Input: part model. Units: mm. Frame: model coordinates. A direction names the side the tool comes from. Coordinates: 2 decimals unless noted, no trailing zeros. Write each loop counter-clockwise with the first axis right and the second up, starting at its lowest first coordinate (ties: lowest second). Pieces come first, ordered by that corner, then holes. Notation, with made-up numbers: (36, 85.5) - (93, 85.5) arc R33 cw to (93, 121.5) - close; hole circle Ø8 at (60.5, 28.5). An arc over 180 degrees is marked (long way). Use CSV: the item, a comma, the result in double quotes.
```python
from build123d import *

# Parameters (mm, degrees)
SKETCH_2_W          = 85.8
SKETCH_2_H          = 85.8
SKETCH_2_R          = 6
EXTRUDE_1_DEPTH     = 13.5
FILLET_1_R          = 10
SKETCH_3_R          = 10
CUT_EXTRUDE_1_DEPTH = 65.366683929


with BuildPart() as part:
    # 草图1 → 旋转1 (revolve)
    with BuildSketch(Plane.XY, mode=Mode.PRIVATE) as revolve_1_sk:
        Polygon((10, 30), (14.5, 30), (14.5, 20), (23, 20), (23, 21.5), (28, 21.5), (28, 3.5), (14.5, 3.5), (14.5, 0), (10, 0), align=None)
    revolve(revolve_1_sk.sketch.rotate(Axis((0, 50.942477876, 0), (0, -1, 0)), 90), axis=Axis((0, 50.942477876, 0), (0, -1, 0)))

    # 草图2 → 凸台-拉伸1 (add)
    with BuildSketch(Plane(origin=(0, -5, 0), x_dir=(1, 0, 0), z_dir=(0, 1, 0))):
        Rectangle(SKETCH_2_W, SKETCH_2_H)
        with Locations(Location((-31.75, 31.75, 0), (0, 0, 270))):
            Circle(SKETCH_2_R, mode=Mode.SUBTRACT)
        with Locations(Location((31.75, 31.75, 0), (0, 0, 270))):
            Circle(SKETCH_2_R, mode=Mode.SUBTRACT)
        with Locations(Location((31.75, -31.75, 0), (0, 0, 270))):
            Circle(SKETCH_2_R, mode=Mode.SUBTRACT)
        with Locations(Location((-31.75, -31.75, 0), (0, 0, 270))):
            Circle(SKETCH_2_R, mode=Mode.SUBTRACT)
    extrude(amount=EXTRUDE_1_DEPTH)

    # 圆角1
    fillet_1_edges = [part.edges().sort_by_distance(p)[0] for p in [
        (42.9, 1.75, 42.9),
        (42.9, 1.75, -42.9),
        (-42.9, 1.75, -42.9),
        (-42.9, 1.75, 42.9),
    ]]
    fillet(fillet_1_edges, radius=FILLET_1_R)

    # 草图3 → 切除-拉伸1 (cut, through all)
    with BuildSketch(Plane(origin=(0, 8.5, 0), x_dir=(1, 0, 0), z_dir=(0, 1, 0))):
        with Locations(Location((0, 0, 0), (0, 0, 270))):
            Circle(SKETCH_3_R)
    extrude(amount=-CUT_EXTRUDE_1_DEPTH, mode=Mode.SUBTRACT)


solid = part.part
```
(1) Pin query (flat end, axial travel): pin 1 Ø1.5 at (y, z) = (18.5, 12.5) entering from +X; pin 2 Ø3 at (y, z) = (21, -2) entering from -X; pin 3 Ø15.5 at (x, z) = (31.75, 31.75) entering from +Y. Return the tip coordinate at first contact, or that it passes through.
Check values:
pin 1,"x = 25.42"
pin 2,"x = -28"
pin 3,"y = 8.5"
(2) Cut plane C-C on x = -31.75. Return loops of the section in (y, z).
Check values:
outline,"(-5, -42.9) - (8.5, -42.9) - (8.5, -37.75) - (-5, -37.75) - close; (-5, -25.75) - (8.5, -25.75) - (8.5, 25.75) - (-5, 25.75) - close; (-5, 37.75) - (8.5, 37.75) - (8.5, 42.9) - (-5, 42.9) - close"
(3) Draft query along Z for faces 1 (the cylindrical face through (28.1, 1.66, -36.51)), 2 (the cylindrical face through (39.89, 1.84, -40.05)), 3 (the flat face through (0, 2, 42.9)). Return one class per face: pulls with the +Z half, pulls with the -Z half, needs draft (parallel to the pull), parting line crosses it, or undercut.
Check values:
face 1,"undercut"
face 2,"pulls with the -Z half"
face 3,"pulls with the +Z half"
(4) Reachability of faces 4 (the cylindrical face through (24.84, 14.91, 12.92)), 5 (the cylindrical face through (28.1, 1.66, 26.99)) from +Z, -Z, +X, -X, +Y, -Y: full face, straight path, thin tool, end or side. Return the list, or none.
Check values:
face 4,"+Y"
face 5,"+Y, -Y"
(5) Cut plane D-D on z = 29.5. Return loops of the section in (x, y), and give its area (3 significant figures).
Check values:
outline,"(-42.9, -5) - (-37.31, -5) - (-37.31, 8.5) - (-42.9, 8.5) - close; (-26.19, -5) - (26.19, -5) - (26.19, 8.5) - (-26.19, 8.5) - close; (37.31, -5) - (42.9, -5) - (42.9, 8.5) - (37.31, 8.5) - close"
area,"858 mm^2"
(6) Cut plane A-A on z = 0. Return loops of the section in (x, y), and give its area (3 significant figures).
Check values:
outline,"(-42.9, -5) - (-10, -5) - (-10, 30) - (-14.5, 30) - (-14.5, 20) - (-23, 20) - (-23, 21.5) - (-28, 21.5) - (-28, 8.5) - (-42.9, 8.5) - close; (10, -5) - (42.9, -5) - (42.9, 8.5) - (28, 8.5) - (28, 21.5) - (23, 21.5) - (23, 20) - (14.5, 20) - (14.5, 30) - (10, 30) - close"
area,"1,410 mm^2"
(7) Ray query, probe 1 along X at (y, z) = (3, -31.75); probe 2 along X at (y, z) = (20.55, 0); probe 3 along Z at (x, y) = (-32.5, 5.5). Return the intervals inside material, ascending. Write a range as from..to.
Check values:
probe 1,"-42.9..-37.75, -25.75..25.75, 37.75..42.9"
probe 2,"-28..-23, -14.5..-10, 10..14.5, 23..28"
probe 3,"-42.9..-37.7, -25.8..25.8, 37.7..42.9"
(8) Cut plane B-B on y = 5.5. Return loops of the section in (x, z).
Check values:
outline,"(-42.9, -32.9) arc R10 ccw to (-32.9, -42.9) - (32.9, -42.9) arc R10 ccw to (42.9, -32.9) - (42.9, 32.9) arc R10 ccw to (32.9, 42.9) - (-32.9, 42.9) arc R10 ccw to (-42.9, 32.9) - close; hole circle Ø12 at (-31.75, -31.75); hole circle Ø12 at (-31.75, 31.75); hole circle Ø20 at (0, 0); hole circle Ø12 at (31.75, -31.75); hole circle Ø12 at (31.75, 31.75)"
